Input: dimensioned drawing with shaded views. Units: mm. Origin: part minimum x, y, z. A direction names the side the tool comes from. Round coordinates to 2 decimals unless told otherwise and drop trailing zeros. Order: outer loops, then holes, each group sorted by start corner. A loop starts at its lowest first (then second) coordinate and runs counter-clockwise, first axis right, second up.
Item 1: Cut plane D-D on z = 7. Output: boundary loops of the cut face in (x, y) (1 decimal).
Item 2: Line query: L1, parallel to Y at x = 3.54, z = 2.4; L2, parallel to Y at x = 8.25, z = 14 (1 decimal). Output: solid intervals per line, ascending.
Item 3: Reachability of the marked faces 1, 2, 3, 4 and 5 from +Z, -Z, +X, -X, +Y, -Y: full face, straight path, thin tool, end or side. Return the list, or none.
Item 4: Mould query, pull axis X, two halves, no side actions, for the marked faces 6, 7 and 8. Classes: released by +X, released by -X, zero draft, split by the parting line, or undercut.
Item 5: Cut plane B-B on z = 9.5. Output: boundary loops of the cut face in (x, y) (1 decimal).
Item 6: First-contact query: pin 1 (1.5 mm diameter, centred on x = 7, z = 12, fed in from +Y) (3 decimals); pin 2 (8 mm diameter, centred on y = 9.5, z = 10, fed in from -X); pin 3 (8 mm diameter, centred on x = 11.5, y = 11.5, fed in from +Z) (3 decimals); pin 4 (6 mm diameter, centred on x = 8, z = 7.5, fed in from -Y). Flat tips, straight axial feed; report the tip coordinate or a pass-through.
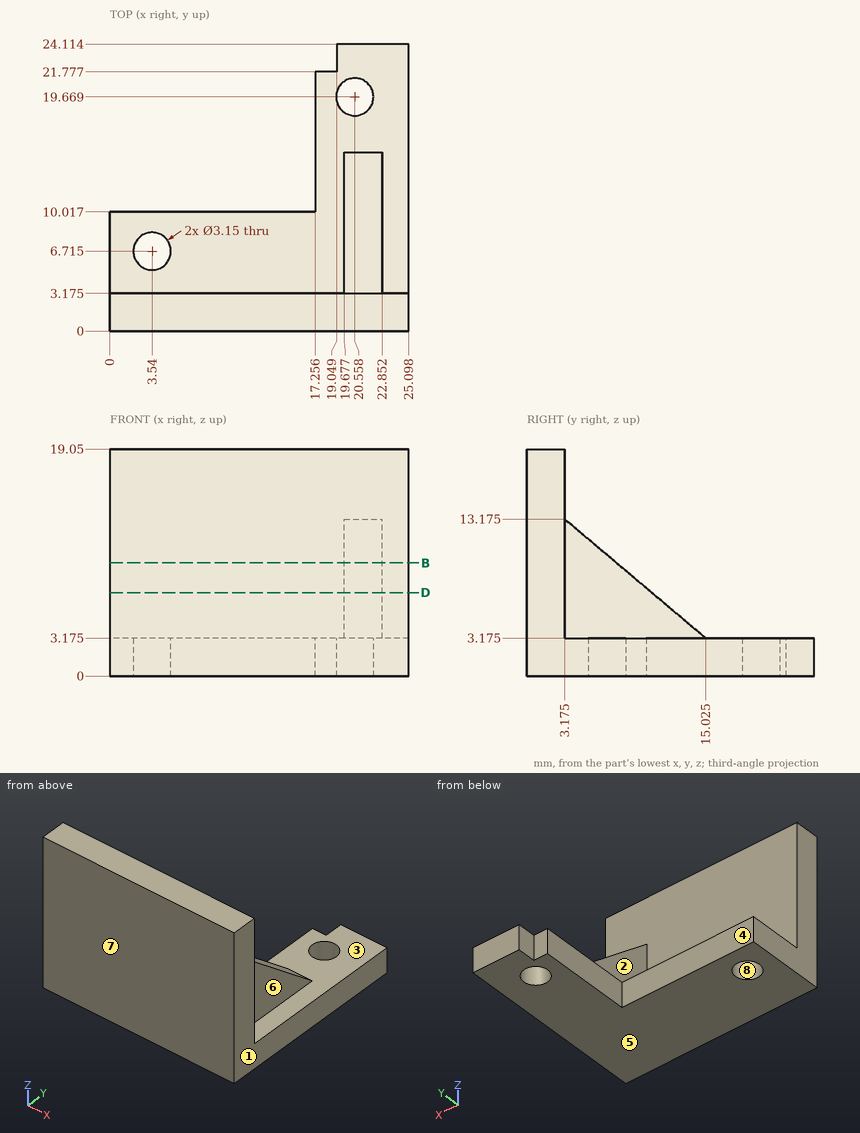
From the geometry:
1. outline: (0, 0) - (25.1, 0) - (25.1, 3.2) - (22.9, 3.2) - (22.9, 10.5) - (19.7, 10.5) - (19.7, 3.2) - (0, 3.2) - close
2. L1: y = 0 to 5.14, 8.29 to 10.02
2. L2: y = 0 to 3.2
3. face 1: +Z, -Z, +X, +Y, -Y
3. face 2: +Z, -X, +Y
3. face 3: +Z, +Y
3. face 4: +Z, -Z, -X, +Y
3. face 5: -Z, +X, -X, +Y, -Y
4. face 6: released by +X
4. face 7: zero draft
4. face 8: undercut
5. outline: (0, 0) - (25.1, 0) - (25.1, 3.2) - (22.9, 3.2) - (22.9, 7.5) - (19.7, 7.5) - (19.7, 3.2) - (0, 3.2) - close
6. pin 1: stops at y = 3.175
6. pin 2: stops at x = 19.68
6. pin 3: stops at z = 3.175
6. pin 4: stops at y = 0
